Geometry: final body of the model. Coordinates: model frame, mm. Coordinates: 2 decimals unless noted, no trailing zeros. Order: outer loops, then holes, each group sorted by start corner. A loop starts at its lowest first (then second) coordinate and runs counter-clockwise, first axis right, second up. Notation, with made-up numbers: (70.25, 42.25) - (77.25, 42.25) arc R15 cw to (77.25, 58.25) - close; hole circle Ø5 at (81.25, 65.5). An arc over 180 degrees is marked (long way). Use a Markdown table: item, result. Add a question column.
Autodesk Inventor part; units mm, degrees
ref_plane "Work Plane1" through (0, 80, 0) normal (0, -1, 0) x (1, 0, 0)
ref_plane "YZ Plane" through (0, 0, 0) normal (1, 0, 0) x (0, 1, 0)
ref_plane "XZ Plane" through (0, 0, 0) normal (0, 1, 0) x (-1, 0, 0)
sketch "Sketch1" plane through (0, 0, 0) normal (0, 1, 0) x (-1, 0, 0)
  line L0 (-75.875, 178) -> (75.875, 178)
  line L1 (75.875, 178) -> (75.875, -178)
  line L2 (75.875, -178) -> (-75.875, -178)
  line L3 (-75.875, -178) -> (-75.875, 178)
  line L4 (-75.875, 178) -> (75.875, -178) construction
  line L5 (75.875, 178) -> (-75.875, -178) construction
  circle A0 centre (67, 170.5) radius 4
  circle A1 centre (-67, 170.5) radius 4
  circle A2 centre (-67, -170.5) radius 4
  circle A3 centre (67, -170.5) radius 4
  line L6 (67, 170.5) -> (-67, 170.5) construction
  line L7 (75.875, 178) -> (67, 170.5) construction
  line L8 (-67, 170.5) -> (-75.875, 178) construction
  line L9 (67, -170.5) -> (67, 170.5) construction
  line L10 (67, -170.5) -> (-67, -170.5) construction
  line L11 (-67, -170.5) -> (-75.875, -178) construction
  line L12 (67, -170.5) -> (75.875, -178) construction
  point P0 (0, 0)
  dimension "d0" = 151.75
  dimension "d1" = 356
  dimension "d11" = 8
  dimension "d12" = 134
  dimension "d13" = 7.5
extrude "Extrusion1" add sketch "Sketch1" along normal blind 108
sketch "Sketch2" plane through (0, 108, 0) normal (0, 1, 0) x (1, 0, 0)
  line L0 (-75.875, -178) -> (75.875, -178)
  line L1 (75.875, 178) -> (-75.875, 178)
  line L2 (-32.875, 178) -> (-32.875, 136.5)
  line L3 (-32.875, 136.5) -> (-9.375, 136.5)
  line L4 (-9.375, 136.5) -> (-9.375, 178)
  line L5 (-32.875, -178) -> (-32.875, -136.5)
  line L6 (-32.875, -136.5) -> (-9.375, -136.5)
  line L7 (-9.375, -136.5) -> (-9.375, -178)
  circle A0 centre (-21.125, -153) radius 3
  circle A1 centre (-21.125, 153) radius 3
  line L8 (-32.875, 178) -> (-21.125, 153) construction
  line L9 (-21.125, 153) -> (-9.375, 178) construction
  line L10 (-32.875, -178) -> (-21.125, -153) construction
  line L11 (-21.125, -153) -> (-9.375, -178) construction
  point P0 (0, 0)
  dimension "d4" = 43
  dimension "d5" = 23.5
  dimension "d6" = 41.5
  dimension "d19" = 6
  dimension "d20" = 25
extrude "Extrusion2" cut sketch "Sketch2" against normal blind 10
sketch "Sketch3" plane through (0, 108, 0) normal (0, 1, 0) x (1, 0, 0)
  line L0 (-32.875, -178) -> (-32.875, -136.5)
  line L1 (-75.875, -178) -> (-32.875, -178)
  line L2 (-31.0347, 131.2602) -> (-10.3663, 131.2602) construction
  line L3 (-10.3663, 131.2602) -> (-10.3663, 113.395) construction
  line L4 (-10.3663, 113.395) -> (-31.0347, 113.395) construction
  line L5 (-31.0347, 113.395) -> (-31.0347, 131.2602) construction
  line L6 (-13.1255, 122.3299) -> (-19.9002, 122.3299)
  line L7 (-19.9002, 122.3299) -> (-19.9002, 115.5552)
  line L8 (-19.9002, 115.5552) -> (-22.1369, 115.5552)
  line L9 (-22.1369, 115.5552) -> (-22.1369, 122.3299)
  line L10 (-22.1369, 122.3299) -> (-28.9116, 122.3299)
  line L11 (-28.9116, 122.3299) -> (-28.9116, 124.4855)
  line L12 (-28.9116, 124.4855) -> (-22.1369, 124.4855)
  line L13 (-22.1369, 124.4855) -> (-22.1369, 131.2602)
  line L14 (-22.1369, 131.2602) -> (-19.9002, 131.2602)
  line L15 (-19.9002, 131.2602) -> (-19.9002, 124.4855)
  line L16 (-19.9002, 124.4855) -> (-13.1255, 124.4855)
  line L17 (-13.1255, 124.4855) -> (-13.1255, 122.3299)
  point P0 (0, 0)
  point P1 (-32.875, 178)
  point P2 (-75.875, 178)
  point P3 (-32.875, 136.5)
extrude "Extrusion3" cut sketch "Sketch3" against normal blind 1
ref_plane "Work Plane1" through (0, 80, 0) normal (0, -1, 0) x (1, 0, 0)
sketch "Sketch4" plane through (0, 108, 0) normal (0, 1, 0) x (1, 0, 0)
  line L0 (-75.875, -178) -> (-32.875, -178)
  line L1 (-75.875, 178) -> (-75.875, -178)
  line L2 (-9.375, -178) -> (75.875, -178)
  line L3 (75.875, -178) -> (75.875, 178)
  line L4 (75.875, 178) -> (-9.375, 178)
  line L5 (-32.875, 178) -> (-75.875, 178)
  line L6 (-75.875, 163.5) -> (-54.875, 163.5)
  line L7 (-54.875, 163.5) -> (-54.875, 178)
  line L8 (54.875, 178) -> (54.875, 163.5)
  line L9 (54.875, 163.5) -> (75.875, 163.5)
  line L10 (54.875, -178) -> (54.875, -163.5)
  line L11 (54.875, -163.5) -> (75.875, -163.5)
  line L12 (-54.875, -178) -> (-54.875, -163.5)
  line L13 (-54.875, -163.5) -> (-75.875, -163.5)
  point P0 (0, 0)
  dimension "d14" = 327
  dimension "d15" = 21
extrude "Extrusion4" cut sketch "Sketch4" against normal up to surface (28 mm away)
sketch "Sketch6" plane through (75.875, 0, 178) normal (1, 0, 0) x (0, 0, -1)
  line L0 (0, 80) -> (0, 108)
  line L1 (0, 108) -> (14.5, 108)
  line L2 (341.5, 108) -> (356, 108)
  line L3 (356, 108) -> (356, 80)
  line L4 (356, 0) -> (0, 0) construction
  line L5 (341.5, 108) -> (341.5, 80)
  line L6 (14.5, 108) -> (14.5, 80)
  line L7 (0, 91) -> (14.5, 91)
  line L8 (341.5, 91) -> (356, 91)
  point P0 (178, 0)
  dimension "d24" = 91
extrude "Extrusion6" cut sketch "Sketch6" against normal up to surface (151.75 mm away)
properties part number "47Ah-FoMoCo"
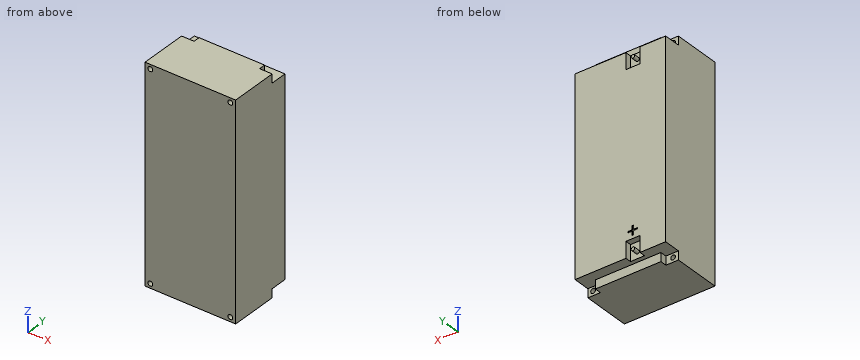
1) First-contact query: pin 1 (11.5 mm diameter, centred on x = -61, z = -172, fed in from +Y); pin 2 (3 mm diameter, centred on x = -25, y = 102.5, fed in from +Z); pin 3 (16 mm diameter, centred on x = 61, z = -172, fed in from +Y). Flat tips, straight axial feed; report the tip coordinate or a pass-through.
2) Line query: line 1 (Z direction, x = -67, y = 31); line 2 (X direction, y = 43, z = 170) (3 decimals); line 3 (Y direction, x = -17, z = -124). Output: solid intervals per line, ascending. Write a range as from..to.
3) Section query A-A (x = 67). Return the cut outline in (y, z), and give its area (3 significant figures).
4) Section query B-B (z = -170.5). Return the cut outline in (x, y) (3 decimals), and give its area (3 significant figures).
From the geometry:
| question | item | result |
|---|---|---|
| 1 | pin 1 | stops at y = 80 |
| 1 | pin 2 | stops at z = 154.83 |
| 1 | pin 3 | stops at y = 91 |
| 2 | line 1 | z = -178..-174.5, -166.5..166.5, 174.5..178 |
| 2 | line 2 | x = -75.875..-70.969, -63.031..63.031, 70.969..75.875 |
| 2 | line 3 | y = 0..107 |
| 3 | outline | (0, -178) - (80, -178) - (80, -174.5) - (0, -174.5) - close; (0, -166.5) - (80, -166.5) - (80, -163.5) - (108, -163.5) - (108, 163.5) - (80, 163.5) - (80, 166.5) - (0, 166.5) - close; (0, 174.5) - (80, 174.5) - (80, 178) - (0, 178) - close |
| 3 | area | 36,400 mm^2 |
| 4 | outline | (-75.875, 0) - (-71, 0) - (-71, 80) - (-75.875, 80) - close; (-63, 0) - (63, 0) - (63, 80) - (54.875, 80) - (54.875, 91) - (-54.875, 91) - (-54.875, 80) - (-63, 80) - close; (71, 0) - (75.875, 0) - (75.875, 80) - (71, 80) - close |
| 4 | area | 12,100 mm^2 |
